Could you check a few things on this model? Use its own coordinates, in mm. Face numbers are marked on the shaded views. A direction names the side the tool comes from. Give positions to 0.01 mm unless a question says otherwise; leave off trailing zeros. Order: outer loops, then holes, each group sorted by start corner. A loop starts at its lowest first (then second) coordinate and runs counter-clockwise, first axis right, second up. Notation, with made-up numbers: M 69.25,18.5 L 120.25,18.5 A11 ccw 120.25,27.5 Z; hole C 18.5,-1 d1. An arc over 180 degrees is marked long. Use a Markdown table: item, result. Add a question column.
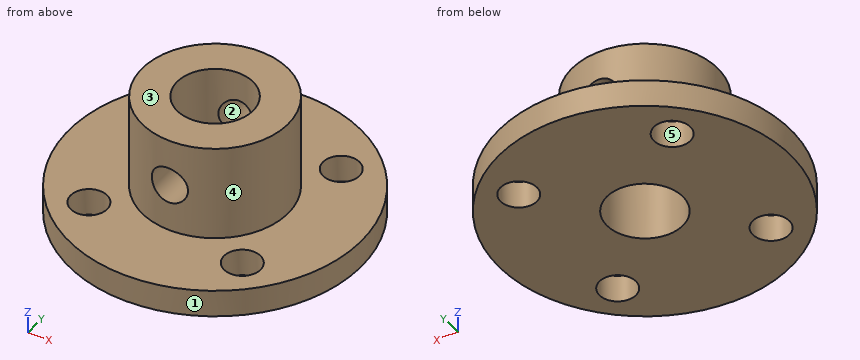
Autodesk Inventor part; units mm, degrees
ref_plane "YZ Plane" through (0, 0, 0) normal (1, 0, 0) x (0, 1, 0)
ref_plane "XZ Plane" through (0, 0, 0) normal (0, 1, 0) x (-1, 0, 0)
ref_plane "XY Plane" through (0, 0, 0) normal (0, 0, 1) x (1, 0, 0)
sketch "Base" plane through (0, 0, 0) normal (0, 0, 1) x (1, 0, 0)
  circle A0 centre (0, 0) radius 4.165
  circle A1 centre (0, 0) radius 8
  circle A2 centre (0, 0) radius 16
  line L0 (-8.4853, 8.4853) -> (8.4853, 8.4853) construction
  line L1 (8.4853, 8.4853) -> (8.4853, -8.4853) construction
  line L2 (8.4853, -8.4853) -> (-8.4853, -8.4853) construction
  line L3 (-8.4853, -8.4853) -> (-8.4853, 8.4853) construction
  circle A3 centre (0, 0) radius 13.4763 construction
  circle A4 centre (0, 0) radius 14 construction
  circle A5 centre (8.4853, 8.4853) radius 2
  circle A6 centre (8.4853, -8.4853) radius 2
  circle A7 centre (-8.4853, -8.4853) radius 2
  circle A8 centre (-8.4853, 8.4853) radius 2
  dimension "d0" = 8.33
  dimension "d1" = 16
  dimension "d2" = 32
  dimension "d3" = 2.5237
  dimension "d4" = 2
  dimension "d5" = 4
extrude "BaseFeature" add sketch "Base" against normal blind 3 contours A1 | A2
extrude "MountFeature" add sketch "Base" along normal blind 10.5 contours A1
sketch "SetScrewHole" plane through (0, 0, 0) normal (0, 1, 0) x (-1, 0, 0)
  circle A0 centre (0, 5.25) radius 2
  line L0 (8, 10.5) -> (-8, 10.5) construction
  line L1 (-8, 0) -> (8, 0) construction
  line L2 (-4.165, 10.5) -> (4.165, 10.5)
  line L3 (0, 10.5) -> (0, 0) construction
  dimension "d10" = 4
extrude "SetScrewHoleFeature" cut sketch "SetScrewHole" along normal through all both and the other way through all
properties part number "Hub8mm"
1) Please list where these lines run through material, in increasing order: line 1 (X direction, y = 7, z = -1.25); line 2 (Z direction, x = 9, y = 2); line 3 (Y direction, x = 2, z = 7.25). Write a range as from..to.
2) Suppose I cut it at B-B on x = 0. Please give me the cut outline in (y, z) (3 decimals), and give its area (3 significant figures).
3) Suppose I cut it at C-C on y = 0. Please give me the cut outline in (x, z) (3 decimals).
4) Suppose I cut it at A-A on y = 7. Please give me the cut outline in (x, z), and give its area (3 significant figures).
5) Suppose I cut it at D-D on z = 5.25. Please give me the cut outline in (x, y) (3 decimals).
6) For the marked faces 4 and 5, which set-ups out of +Z, -Z, +X, -X, +Y, -Y let a thin tool reach every point of the face, with its end or its side?
7) For pin 1 (6 mm diameter, centred on y = -2, z = 2.5, fed in from -X); pin 2 (4.5 mm diameter, centred on x = 0, z = 5.25, fed in from -Y); pin 3 (6.5 mm diameter, centred on x = 8.49, y = 8.49, fed in from +Z), each with a flat end and sliding along its axis, tell me the tip position at first contact or that it passes through.
8) We'd pull the mould along X, two halves only. Please class the marked faces 1, 2 and 3: pulls with the +X half, pulls with the -X half, needs draft (parallel to the pull), parting line crosses it, or undercut.
Values found:
| question | item | result |
|---|---|---|
| 1 | line 1 | x = -14.39..-9.82, -7.15..7.15, 9.82..14.39 |
| 1 | line 2 | z = -3..0 |
| 1 | line 3 | y = -7.75..-3.65, 3.65..7.75 |
| 2 | outline | M -16,-3 L -4.165,-3 L -4.165,3.25 L -8,3.25 L -8,0 L -16,0 Z; M -8,7.25 L -4.165,7.25 L -4.165,10.5 L -8,10.5 Z; M 4.165,-3 L 16,-3 L 16,0 L 8,0 L 8,3.25 L 4.165,3.25 Z; M 4.165,7.25 L 8,7.25 L 8,10.5 L 4.165,10.5 Z |
| 2 | area | 121 mm^2 |
| 3 | outline | M -16,-3 L -4.165,-3 L -4.165,10.5 L -8,10.5 L -8,0 L -16,0 Z; M 4.165,-3 L 16,-3 L 16,0 L 8,0 L 8,10.5 L 4.165,10.5 Z |
| 4 | outline | M -14.39,-3 L -9.82,-3 L -9.82,0 L -14.39,0 Z; M -7.15,-3 L 7.15,-3 L 7.15,0 L 3.87,0 L 3.87,10.5 L -3.87,10.5 L -3.87,0 L -7.15,0 Z; M 9.82,-3 L 14.39,-3 L 14.39,0 L 9.82,0 Z; hole C 0,5.25 d4 |
| 4 | area | 139 mm^2 |
| 5 | outline | M -2,-7.746 L -2,-3.653 A4.165 cw -2,3.653 L -2,7.746 A8 ccw Z; M 2,-7.746 A8 ccw 2,7.746 L 2,3.653 A4.165 cw 2,-3.653 Z |
| 6 | face 4 | +Z |
| 6 | face 5 | +Z, -Z |
| 7 | pin 1 | stops at x = -16 |
| 7 | pin 2 | stops at y = -8 |
| 7 | pin 3 | stops at z = 0 |
| 8 | face 1 | parting line crosses it |
| 8 | face 2 | undercut |
| 8 | face 3 | needs draft |
